```python
from build123d import *

# Parameters (mm, degrees)
F1_DEPTH = 1.6


with BuildPart() as f1:
    # F0 (on Top) → F1 (new body)
    with BuildSketch(Plane.XY):
        with BuildLine():
            ThreePointArc((8.7867965644, -8.7867965644), (2.2836140247, -18.519497029), (0, -30))
            ThreePointArc((0, -30), (8.7867965644, -51.2132034356), (30, -60))
            ThreePointArc((30, -60), (41.480502971, -57.7163859753), (51.2132034356, -51.2132034356))
            Line((51.2132034356, -51.2132034356), (40.6066017178, -40.6066017178))
            ThreePointArc((40.6066017178, -40.6066017178), (19.3933982822, -40.6066017178), (19.3933982822, -19.3933982822))
            Line((19.3933982822, -19.3933982822), (8.7867965644, -8.7867965644))
        make_face()
        with BuildLine():
            ThreePointArc((60, -30), (51.2132034356, -8.7867965644), (30, 0))
            ThreePointArc((30, 0), (18.519497029, -2.2836140247), (8.7867965644, -8.7867965644))
            Line((8.7867965644, -8.7867965644), (19.3933982822, -19.3933982822))
            ThreePointArc((19.3933982822, -19.3933982822), (35.7402514855, -16.1418070123), (45, -30))
            ThreePointArc((45, -30), (43.8581929877, -35.7402514855), (40.6066017178, -40.6066017178))
            Line((40.6066017178, -40.6066017178), (51.2132034356, -51.2132034356))
            ThreePointArc((51.2132034356, -51.2132034356), (57.7163859753, -41.480502971), (60, -30))
        make_face()
    extrude(amount=F1_DEPTH)


solid = f1.part
```
Input: part model. Units: mm. Frame: model coordinates. Round coordinates to 2 decimals unless told otherwise and drop trailing zeros. Loops run counter-clockwise (first coordinate to the right, second up) from the corner with the lowest first, then second, coordinate; pieces in that order, holes last. Notation, with made-up numbers: (-33.5, 46.5) -> (-7.5, 46.5) arc R26 cw to (-7.5, 77.5) -> close; hole circle Ø1 at (8.25, -3.5). An arc over 180 degrees is marked (long way). Write each question's results on one line, items separated by ' | '.
1. Section C-C (x = 29). Return loops of the section in (y, z).
Geometry results:
outline: (-59.98, 0) -> (-44.97, 0) -> (-44.97, 1.6) -> (-59.98, 1.6) -> close; (-15.03, 0) -> (-0.02, 0) -> (-0.02, 1.6) -> (-15.03, 1.6) -> close
2. Section D-D (y = -55.5). Return loops of the section in (x, z), and give its area (3 significant figures).
Geometry results:
outline: (14.2, 0) -> (45.8, 0) -> (45.8, 1.6) -> (14.2, 1.6) -> close | area: 50.6 mm2
3. Ray query, line 1 (Y direction, x = 17, z = 0.15); line 2 (Y direction, x = 18, z = 0.75); line 3 (X direction, y = -22, z = 0.8). Return the intervals inside material, ascending. Write a range as from..to.
Geometry results:
line 1: -57.04..-37.48, -22.52..-2.96 | line 2: -57.5..-39, -21..-2.5 | line 3: 1.09..17.31, 42.69..58.91
4. Section A-A (z = 0.35). Return loops of the section in (x, y), and give its area (3 significant figures).
Geometry results:
outline: circle Ø60 at (30, -30); hole circle Ø30 at (30, -30) | area: 2,120 mm2
5. Section B-B (y = -36.5). Return loops of the section in (x, z).
Geometry results:
outline: (0.71, 0) -> (16.48, 0) -> (16.48, 1.6) -> (0.71, 1.6) -> close; (43.52, 0) -> (59.29, 0) -> (59.29, 1.6) -> (43.52, 1.6) -> close
